Autodesk Inventor part; units mm, degrees
ref_plane "YZ Plane" through (0, 0, 0) normal (1, 0, 0) x (0, 1, 0)
ref_plane "XZ Plane" through (0, 0, 0) normal (0, 1, 0) x (-1, 0, 0)
ref_plane "XY Plane" through (0, 0, 0) normal (0, 0, 1) x (1, 0, 0)
sketch "Sketch1" plane through (0, 0, 0) normal (1, 0, 0) x (0, 1, 0)
  line L0 (1250.1265, -201.1417) -> (1330.5832, 0)
  line L1 (0, 0) -> (1330.5832, 0)
  line L2 (0, -220) -> (0, 0)
  line L3 (1222.2722, -220) -> (0, -220)
  arc A0 (1222.2722, -220) -> (1250.1265, -201.1417) centre (1222.2722, -190) ccw
extrude "Extrusion1" add sketch "Sketch1" along normal blind 1.5
properties part number "CARCASA_ALUM_2_FLAT" material "Steel, Mild, Welded"
The model under review builds one solid part; all positions refer to its coordinate system, in mm. Give positions to 0.01 mm unless a question says otherwise; leave off trailing zeros. Write each loop counter-clockwise with the first axis right and the second up, starting at its lowest first coordinate (ties: lowest second). Pieces come first, ordered by that corner, then holes. Notation, with made-up numbers: M -22.75,29.5 L 5.25,29.5 A8 cw 5.25,36.5 Z; hole C 72.25,22.25 d4. An arc over 180 degrees is marked long. Answer in a Markdown table with one row per item.
Item 1: Add section B-B on z = -108. Give the boundary of the cut face in (x, y), plus the area to 3 significant figures.
Check sheet entries:
| item | result |
|---|---|
| outline | M 0,0 L 1.5,0 L 1.5,1287.38 L 0,1287.38 Z |
| area | 1,930 mm2 |
Item 2: Add section A-A on x = 0.6. Give the boundary of the cut face in (y, z).
Check sheet entries:
| item | result |
|---|---|
| outline | M 0,-220 L 1222.27,-220 A30 ccw 1250.13,-201.14 L 1330.58,0 L 0,0 Z |
Item 3: For P1, Ø2, axis at y = 153.5, z = -74.5, coming from the -X side, flat-tipped, find the tip position at first contact; note if it passes through.
Check sheet entries:
| item | result |
|---|---|
| P1 | x = 0 |
Item 4: For line 1 along Y through (x, z) = (1.1, -75); line 2 along Y through (x, z) = (0.4, -45); line 3 along Z through (x, y) = (1, 1245), list the stretches that pass through material, from the lowest coordinate up.
Check sheet entries:
| item | result |
|---|---|
| line 1 | 0 to 1300.58 |
| line 2 | 0 to 1312.58 |
| line 3 | -209.58 to 0 |
